The figure shows three views and two pictorial views of one solid part (mm, origin at its lowest corner). Answer the questions. A direction names the side the tool comes from. Round coordinates to 2 decimals unless told otherwise and drop trailing zeros. Order: outer loops, then holes, each group sorted by start corner. A loop starts at its lowest first (then second) coordinate and runs counter-clockwise, first axis right, second up. Notation, with made-up numbers: (36.5, -35) - (79.5, -35) arc R10 cw to (79.5, -30) - close; hole circle Ø11 at (72, 23.5). An arc over 180 degrees is marked (long way). Use CSV: the item, a comma, the result in double quotes.
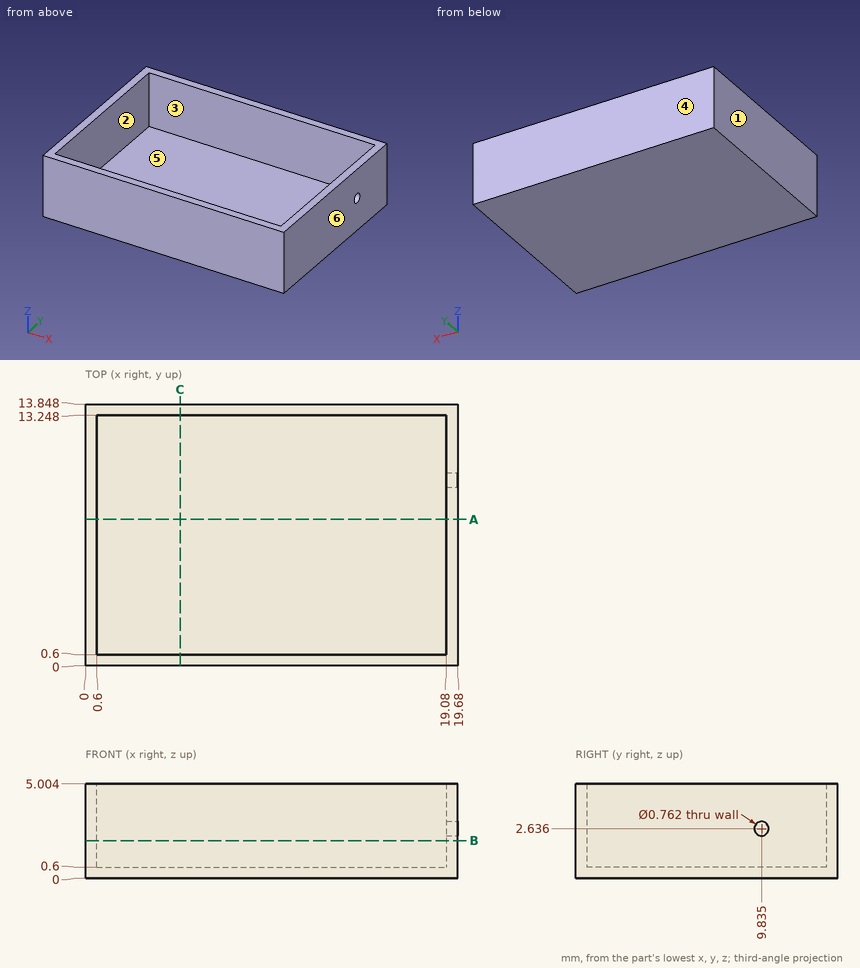
(1) For the marked faces 1 and 2, determine the directions among +Z, -Z, +X, -X, +Y, -Y from which every point of the face is accessible in a straight line to the end or side of a thin tool.
Findings below:
face 1,"+Z, -Z, -X, +Y, -Y"
face 2,"+Z"
(2) Find section A-A (y = 7.75). Determine the outline of the cut face in (x, z).
Findings below:
outline,"(0, 0) - (19.68, 0) - (19.68, 5) - (19.08, 5) - (19.08, 0.6) - (0.6, 0.6) - (0.6, 5) - (0, 5) - close"
(3) Find section B-B (z = 2). Determine the outline of the cut face in (x, y).
Findings below:
outline,"(0, 0) - (19.68, 0) - (19.68, 13.85) - (0, 13.85) - close; hole (0.6, 0.6) - (19.08, 0.6) - (19.08, 13.25) - (0.6, 13.25) - close"
(4) Find the intervals of material crossed by L1, parallel to Y at x = 5.25, z = 4.8; L2, parallel to X at y = 7.25, z = 3.65; L3, parallel to Z at x = 11, y = 3.25, in increasing order. Write a range as from..to.
Findings below:
L1,"y = 0..0.6, 13.25..13.85"
L2,"x = 0..0.6, 19.08..19.68"
L3,"z = 0..0.6"
(5) The mould has two halves that part along X. Classify the marked faces 3, 4, 5 and 6: released by +X, released by -X, zero draft, split by the parting line, or undercut.
Findings below:
face 3,"undercut"
face 4,"zero draft"
face 5,"undercut"
face 6,"released by +X"
(6) Find section C-C (x = 5). Determine the outline of the cut face in (y, z).
Findings below:
outline,"(0, 0) - (13.85, 0) - (13.85, 5) - (13.25, 5) - (13.25, 0.6) - (0.6, 0.6) - (0.6, 5) - (0, 5) - close"
